The listing builds one solid part. Answer for the finished solid, in the listing's coordinates (mm). Face numbers are marked on the shaded views. A direction names the side the tool comes from. Coordinates: 2 decimals unless noted, no trailing zeros. Write each loop counter-clockwise with the first axis right and the second up, starting at its lowest first coordinate (ties: lowest second). Pieces come first, ordered by that corner, then holes.
from build123d import *

# Parameters (mm, degrees)
F0_R     = 76.2
F0_R_2   = 44.45
F1_DEPTH = 2.54
F2_DEPTH = 17.78
F3_DEPTH = 25.4


with BuildPart() as f1:
    # F0 (on Front) → F1 (new body)
    with BuildSketch(Plane.XZ):
        Circle(F0_R)
        Circle(F0_R_2, mode=Mode.SUBTRACT)
    extrude(amount=F1_DEPTH)

    # F0 (on Front) → F2 (join)
    with BuildSketch(Plane.XZ):
        Circle(F0_R_2)
    extrude(amount=F2_DEPTH)

    # F0 (on Front) → F3 (join)
    with BuildSketch(Plane.XZ):
        Circle(F0_R)
        Circle(F0_R_2, mode=Mode.SUBTRACT)
        Circle(F0_R_2)
    extrude(amount=-F3_DEPTH)


solid = f1.part
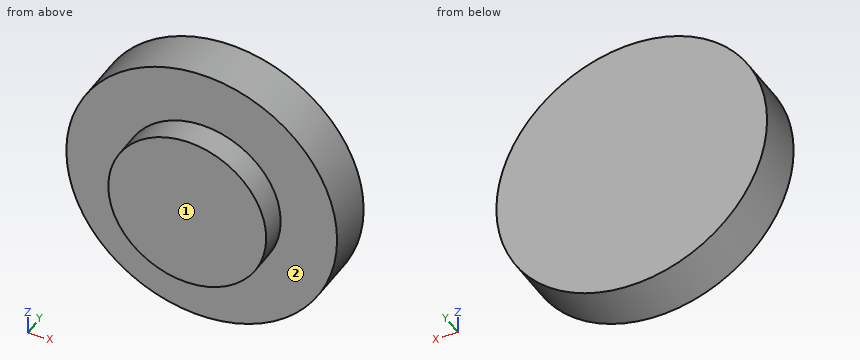
Q1. The part is cut by section A-A, the plane x = 0. Write down the section's boundary in (y, z), then the cut area to 3 significant figures.
Answers below:
outline: (-17.78, -44.45) - (-2.54, -44.45) - (-2.54, -76.2) - (25.4, -76.2) - (25.4, 76.2) - (-2.54, 76.2) - (-2.54, 44.45) - (-17.78, 44.45) - close
area: 5,610 mm2
Q2. The part is cut by section C-C, the plane y = 19. Write down the section's boundary in (x, z).
Answers below:
outline: circle Ø152.4 at (0, 0)
Q3. The part is cut by section D-D, the plane x = 65. Write down the section's boundary in (y, z), then the cut area to 3 significant figures.
Answers below:
outline: (-2.54, -39.77) - (25.4, -39.77) - (25.4, 39.77) - (-2.54, 39.77) - close
area: 2,220 mm2
Q4. Find the intervals of material crossed by probe 1 along Y at (x, z) = (-31, -54); probe 2 along X at (y, z) = (-16, 33); probe 3 along Z at (x, y) = (-3.5, 12), in increasing order.
Answers below:
probe 1: y = -2.54 to 25.4
probe 2: x = -29.78 to 29.78
probe 3: z = -76.12 to 76.12
Q5. The part is cut by section B-B, the plane z = 0. Write down the section's boundary in (x, y), then the cut area to 3 significant figures.
Answers below:
outline: (-76.2, -2.54) - (-44.45, -2.54) - (-44.45, -17.78) - (44.45, -17.78) - (44.45, -2.54) - (76.2, -2.54) - (76.2, 25.4) - (-76.2, 25.4) - close
area: 5,610 mm2
Q6. Given pin 1 (8 mm diameter, centred on x = 18, y = 15.5, fed in from -Z); pin 2 (2 mm diameter, centred on x = -44, z = 26, fed in from -Y); pin 3 (4 mm diameter, centred on y = -3, z = -12, fed in from -X); pin 4 (2 mm diameter, centred on x = 51, z = 58, fed in from +Y), each flat-ended and moving along its own axis, determine where each tip first touches the part or whether it passes through.
Answers below:
pin 1: stops at z = -74.9
pin 2: stops at y = -2.54
pin 3: stops at x = -75.53
pin 4: passes through
Q7. Which of the six approach directions +Z, -Z, +X, -X, +Y, -Y give full straight-line access (tool end or side, diameter ignored) to the marked faces 1 and 2?
Answers below:
face 1: +Z, -Z, +X, -X, -Y
face 2: -Y
